from build123d import *

# Parameters (mm, degrees)
BOSS_EXTRUDE1_DEPTH = 2
SKETCH2_W           = 102
SKETCH2_H           = 37.25
BOSS_EXTRUDE2_DEPTH = 2
SKETCH3_W           = 10.5265
SKETCH3_H           = 3.907167626
CUT_EXTRUDE1_DEPTH  = 2


with BuildPart() as part:
    # Sketch1 → Boss-Extrude1 (new body)
    with BuildSketch(Plane(origin=(0, 0, 0), x_dir=(1, 0, 0), z_dir=(0, 1, 0))):
        with BuildLine():
            Line((51, -21.625), (-51, -21.625))
            ThreePointArc((-51, -21.625), (-53.121320344, -20.746320344), (-54, -18.625))
            Line((-54, -18.625), (-54, 18.625))
            ThreePointArc((-54, 18.625), (-53.121320344, 20.746320344), (-51, 21.625))
            Line((-51, 21.625), (51, 21.625))
            ThreePointArc((51, 21.625), (53.121320344, 20.746320344), (54, 18.625))
            Line((54, 18.625), (54, -18.625))
            ThreePointArc((54, -18.625), (53.121320344, -20.746320344), (51, -21.625))
        make_face()
    extrude(amount=BOSS_EXTRUDE1_DEPTH)

    # Sketch2 → Boss-Extrude2 (add)
    with BuildSketch(Plane(origin=(0, 2, 0), x_dir=(1, 0, 0), z_dir=(0, 1, 0))):
        with BuildLine():
            Line((51, -19.625), (-51, -19.625))
            ThreePointArc((-51, -19.625), (-51.707106781, -19.332106781), (-52, -18.625))
            Line((-52, -18.625), (-52, 18.625))
            ThreePointArc((-52, 18.625), (-51.707106781, 19.332106781), (-51, 19.625))
            Line((-51, 19.625), (51, 19.625))
            ThreePointArc((51, 19.625), (51.707106781, 19.332106781), (52, 18.625))
            Line((52, 18.625), (52, -18.625))
            ThreePointArc((52, -18.625), (51.707106781, -19.332106781), (51, -19.625))
        make_face()
        Rectangle(SKETCH2_W, SKETCH2_H, mode=Mode.SUBTRACT)
    extrude(amount=BOSS_EXTRUDE2_DEPTH)

    # Sketch3 → Cut-Extrude1 (cut)
    with BuildSketch(Plane.XY.offset(19.625)):
        with Locations((-43.32145, 3.953583813)):
            Rectangle(SKETCH3_W, SKETCH3_H)
    extrude(amount=-CUT_EXTRUDE1_DEPTH, mode=Mode.SUBTRACT)


solid = part.part
The listing builds one solid part. Answer for the finished solid, in the listing's coordinates (mm). A direction names the side the tool comes from. Give positions to 0.01 mm unless a question says otherwise; leave off trailing zeros. Write each loop counter-clockwise with the first axis right and the second up, starting at its lowest first coordinate (ties: lowest second). Pieces come first, ordered by that corner, then holes. Notation, with made-up numbers: (-13.5, -40) -> (1.5, -40) arc R11 cw to (1.5, -29) -> close; hole circle Ø5 at (87, 76). An arc over 180 degrees is marked (long way). Use a Markdown table: item, result.
(1) Determine the mould class of faces 4 (the flat face through (1, 2, 0)), 5 (the flat face through (51, 3, 0)), 6 (the flat face through (-52, 3, 0)), 7 (the flat face through (-1, 1, -21.625)) for opening direction X: released by +X, released by -X, zero draft, split by the parting line, or undercut.
Return value:
| item | result |
|---|---|
| face 4 | undercut |
| face 5 | undercut |
| face 6 | released by -X |
| face 7 | zero draft |
(2) For faces 1 (the flat face through (7, 3, 19.625)), 2 (the flat face through (-50, 3, 18.625)), 3 (the flat face through (52, 3, 0)), determine the directions among +Z, -Z, +X, -X, +Y, -Y from which every point of the face is accessible in a straight line to the end or side of a thin tool.
Return value:
| item | result |
|---|---|
| face 1 | +Z, +X, -X, +Y |
| face 2 | +Y |
| face 3 | +Z, -Z, +X, +Y |
(3) Section B-B, the plane z = 17 is taken. Determine the outline of the cut face in (x, y), then the cut area to 3 significant figures.
Return value:
| item | result |
|---|---|
| outline | (-54, 0) -> (54, 0) -> (54, 2) -> (52, 2) -> (52, 4) -> (51, 4) -> (51, 2) -> (-51, 2) -> (-51, 4) -> (-52, 4) -> (-52, 2) -> (-54, 2) -> close |
| area | 220 mm2 |
(4) Section D-D, the plane x = 11 is taken. Determine the outline of the cut face in (y, z) (3 decimals).
Return value:
| item | result |
|---|---|
| outline | (0, -21.625) -> (2, -21.625) -> (2, -19.625) -> (4, -19.625) -> (4, -18.625) -> (2, -18.625) -> (2, 18.625) -> (4, 18.625) -> (4, 19.625) -> (2, 19.625) -> (2, 21.625) -> (0, 21.625) -> close |
(5) Find the intervals of material crossed by probe 1 along X at (y, z) = (3.25, -1.5); probe 2 along Z at (x, y) = (-17, 3.8) (3 decimals); probe 3 along Y at (x, z) = (3, 3), in increasing order. Write a range as from..to.
Return value:
| item | result |
|---|---|
| probe 1 | -52..-51, 51..52 |
| probe 2 | -19.625..-18.625, 18.625..19.625 |
| probe 3 | 0..2 |
(6) Section C-C, the plane x = -41 is taken. Determine the outline of the cut face in (y, z) (3 decimals), then the cut area to 3 significant figures.
Return value:
| item | result |
|---|---|
| outline | (0, -21.625) -> (2, -21.625) -> (2, -19.625) -> (4, -19.625) -> (4, -18.625) -> (2, -18.625) -> (2, 21.625) -> (0, 21.625) -> close |
| area | 88.5 mm2 |
(7) Flat-ended cylindrical pins translate along their axes: P1, Ø0.6, axis at y = 2.5, z = 2.5, coming from the +X side; P2, Ø1.6, axis at x = -10, y = 3.5, coming from the -Z side (3 decimals); P3, Ø0.6, axis at x = 2.5, y = 2.5, coming from the +Z side (3 decimals); P4, Ø4, axis at x = -12, z = -9.5, coming from the -Y side. Find the tip coordinate at first contact, or state that the pin passes through.
Return value:
| item | result |
|---|---|
| P1 | x = 52 |
| P2 | z = -19.625 |
| P3 | z = 19.625 |
| P4 | y = 0 |
(8) Section A-A, the plane y = 2.7 is taken. Determine the outline of the cut face in (x, z) (3 decimals).
Return value:
| item | result |
|---|---|
| outline | (-52, -18.625) arc R1 ccw to (-51, -19.625) -> (51, -19.625) arc R1 ccw to (52, -18.625) -> (52, 18.625) arc R1 ccw to (51, 19.625) -> (-38.058, 19.625) -> (-38.058, 18.625) -> (51, 18.625) -> (51, -18.625) -> (-51, -18.625) -> (-51, 18.625) -> (-48.585, 18.625) -> (-48.585, 19.625) -> (-51, 19.625) arc R1 ccw to (-52, 18.625) -> close |
